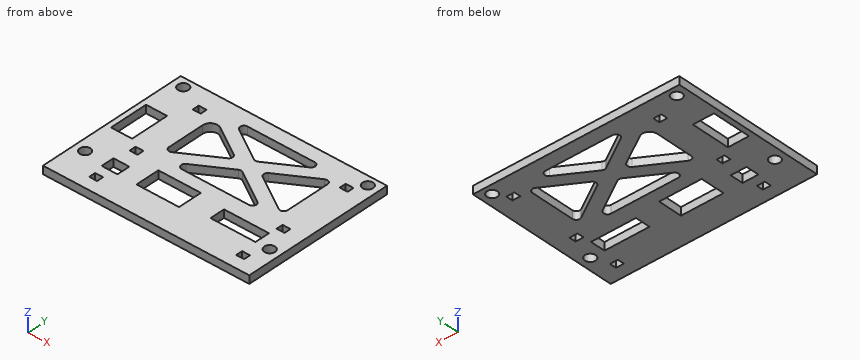
from build123d import *

# Parameters (mm, degrees)
SKETCH1_W              = 41.275
SKETCH1_H              = 25.4
SKETCH1_R              = 1.0541
SKETCH1_H_2            = 5.08
BOSS_EXTRUDE1_DEPTH    = 1.5875
ATTACHMENT_HOLES_REACH = 34.766
SKETCH3_W              = 1.5875
SKETCH3_H              = 1.3208
SKETCH2_W              = 8.509
SKETCH2_H              = 4.826
SKETCH2_W_2            = 4.22
SKETCH2_H_2            = 7.75
SKETCH2_W_3            = 3.175
SKETCH2_H_3            = 2.6162
SKETCH2_W_4            = 9
SKETCH2_H_4            = 2.985879982
CUT_EXTRUDE1_DEPTH     = 1.5875
FILLET8_R              = 0.762
FILLET9_R              = 1.524


with BuildPart() as part:
    # Sketch1 → Boss-Extrude1 (new body)
    # profile 1 of 2: a face of its own
    with BuildSketch(Plane.XY):
        with Locations((0, 12.7)):
            Rectangle(SKETCH1_W, SKETCH1_H)
        with Locations((-18.4658, 1.8415)):
            Circle(SKETCH1_R, mode=Mode.SUBTRACT)
        with Locations((18.4658, 1.8415)):
            Circle(SKETCH1_R, mode=Mode.SUBTRACT)
        with Locations((-18.4658, 23.5585)):
            Circle(SKETCH1_R, mode=Mode.SUBTRACT)
        with Locations((18.4658, 23.5585)):
            Circle(SKETCH1_R, mode=Mode.SUBTRACT)
    # profile 2 of 2: a face of its own
    with BuildSketch(Plane.XY):
        with Locations((0, -2.54)):
            Rectangle(SKETCH1_W, SKETCH1_H_2)
    extrude(amount=BOSS_EXTRUDE1_DEPTH)

    # Sketch3 → Attachment Holes (cut, up to next)
    with BuildSketch(Plane(origin=(0, 0, 0), x_dir=(-1, 0, 0), z_dir=(0, 0, -1)), mode=Mode.PRIVATE) as attachment_holes_sk1:
        with Locations((-16.54175, 20.992155968)):
            Rectangle(SKETCH3_W, SKETCH3_H)
    attachment_holes_tool1 = extrude(attachment_holes_sk1.sketch, amount=-ATTACHMENT_HOLES_REACH, mode=Mode.PRIVATE) & part.part
    # Sketch3 → Attachment Holes (cut, up to next)
    with BuildSketch(Plane(origin=(0, 0, 0), x_dir=(-1, 0, 0), z_dir=(0, 0, -1)), mode=Mode.PRIVATE) as attachment_holes_sk2:
        with Locations((-16.54175, 7.022155968)):
            Rectangle(SKETCH3_W, SKETCH3_H)
    attachment_holes_tool2 = extrude(attachment_holes_sk2.sketch, amount=-ATTACHMENT_HOLES_REACH, mode=Mode.PRIVATE) & part.part
    # Sketch3 → Attachment Holes (cut, up to next)
    with BuildSketch(Plane(origin=(0, 0, 0), x_dir=(-1, 0, 0), z_dir=(0, 0, -1)), mode=Mode.PRIVATE) as attachment_holes_sk3:
        with Locations((-16.54175, -1.918644032)):
            Rectangle(SKETCH3_W, SKETCH3_H)
    attachment_holes_tool3 = extrude(attachment_holes_sk3.sketch, amount=-ATTACHMENT_HOLES_REACH, mode=Mode.PRIVATE) & part.part
    # Sketch3 → Attachment Holes (cut, up to next)
    with BuildSketch(Plane(origin=(0, 0, 0), x_dir=(-1, 0, 0), z_dir=(0, 0, -1)), mode=Mode.PRIVATE) as attachment_holes_sk4:
        with Locations((12.85875, 20.992155968)):
            Rectangle(SKETCH3_W, SKETCH3_H)
    attachment_holes_tool4 = extrude(attachment_holes_sk4.sketch, amount=-ATTACHMENT_HOLES_REACH, mode=Mode.PRIVATE) & part.part
    # Sketch3 → Attachment Holes (cut, up to next)
    with BuildSketch(Plane(origin=(0, 0, 0), x_dir=(-1, 0, 0), z_dir=(0, 0, -1)), mode=Mode.PRIVATE) as attachment_holes_sk5:
        with Locations((12.85875, 7.022155968)):
            Rectangle(SKETCH3_W, SKETCH3_H)
    attachment_holes_tool5 = extrude(attachment_holes_sk5.sketch, amount=-ATTACHMENT_HOLES_REACH, mode=Mode.PRIVATE) & part.part
    # Sketch3 → Attachment Holes (cut, up to next)
    with BuildSketch(Plane(origin=(0, 0, 0), x_dir=(-1, 0, 0), z_dir=(0, 0, -1)), mode=Mode.PRIVATE) as attachment_holes_sk6:
        with Locations((12.85875, -1.918644032)):
            Rectangle(SKETCH3_W, SKETCH3_H)
    attachment_holes_tool6 = extrude(attachment_holes_sk6.sketch, amount=-ATTACHMENT_HOLES_REACH, mode=Mode.PRIVATE) & part.part
    add(attachment_holes_tool1.solids().sort_by_distance((16.54175, 20.992156, 0))[0], mode=Mode.SUBTRACT)
    add(attachment_holes_tool2.solids().sort_by_distance((16.54175, 7.022156, 0))[0], mode=Mode.SUBTRACT)
    add(attachment_holes_tool3.solids().sort_by_distance((16.54175, -1.918644, 0))[0], mode=Mode.SUBTRACT)
    add(attachment_holes_tool4.solids().sort_by_distance((-12.85875, 20.992156, 0))[0], mode=Mode.SUBTRACT)
    add(attachment_holes_tool5.solids().sort_by_distance((-12.85875, 7.022156, 0))[0], mode=Mode.SUBTRACT)
    add(attachment_holes_tool6.solids().sort_by_distance((-12.85875, -1.918644, 0))[0], mode=Mode.SUBTRACT)

    # Sketch2 → Cut-Extrude1 (cut)
    with BuildSketch(Plane.XY.offset(1.5875)):
        Polygon((11.409828794, 8.0735), (1.9685, 13.850842654), (-7.472828794, 8.0735), align=None)
        Polygon((13.843, 21.117092654), (4.401671206, 15.33975), (13.843, 9.562407346), align=None)
        Polygon((-7.472828794, 22.606), (1.9685, 16.828657346), (11.409828794, 22.606), align=None)
        Polygon((-0.464671206, 15.33975), (-9.906, 21.117092654), (-9.906, 9.562407346), align=None)
        with Locations((-2.8993, 3.1205)):
            Rectangle(SKETCH2_W, SKETCH2_H)
        with Locations((-17.4978, 12.709)):
            Rectangle(SKETCH2_W_2, SKETCH2_H_2)
        with Locations((-12.5513, 2.0156)):
            Rectangle(SKETCH2_W_3, SKETCH2_H_3)
        with Locations((11.1858, 3.267239991)):
            Rectangle(SKETCH2_W_4, SKETCH2_H_4)
    extrude(amount=-CUT_EXTRUDE1_DEPTH, mode=Mode.SUBTRACT)

    # Fillet8
    fillet8_edges = [part.edges().sort_by_distance(p)[0] for p in [
        (-7.472828794, 8.0735, 0.79375),
        (1.9685, 13.850842654, 0.79375),
        (11.409828794, 8.0735, 0.79375),
        (4.401671206, 15.33975, 0.79375),
        (13.843, 21.117092654, 0.79375),
        (13.843, 9.562407346, 0.79375),
        (1.9685, 16.828657346, 0.79375),
        (-7.472828794, 22.606, 0.79375),
        (11.409828794, 22.606, 0.79375),
        (-9.906, 9.562407346, 0.79375),
        (-0.464671206, 15.33975, 0.79375),
    ]]
    fillet(fillet8_edges, radius=FILLET8_R)

    # Fillet9
    fillet9_edges = [part.edges().sort_by_distance(p)[0] for p in [
        (-9.906, 21.117092654, 0.79375),
    ]]
    fillet(fillet9_edges, radius=FILLET9_R)


solid = part.part
Here's how the part is built. I have some questions about the finished solid (model axes, mm). Round coordinates to 2 decimals unless told otherwise and drop trailing zeros. Loops run counter-clockwise (first coordinate to the right, second up) from the corner with the lowest first, then second, coordinate; pieces in that order, holes last. Notation, with made-up numbers: M 11.25,-35.75 L 24.25,-35.75 A22 ccw 24.25,-8.75 Z; hole C 52.5,63 d9. An arc over 180 degrees is marked long. Write each question's results on one line, items separated by ' | '. Start each with the question number.
(1) Will these pins go through, and if not, where does the flat tip stop? P1, Ø1, axis at x = 4.5, y = 19.5, coming from the +Z side; P2, Ø3.5, axis at x = -18.47, y = 1.84, coming from the +Z side.
(2) I want a section at B-B (y = 7). Please give me the cut outline in (x, z) (1 decimal).
(3) If I drill on probe 1 along X at (y, z) = (23.5, 1.35); probe 2 along X at (y, z) = (6.5, 0.2) (1 decimal); probe 3 along X at (y, z) = (15, 1.2), over which ranges is the centre line in solid material (lowest first)? Write a range as from..to.
(4) I want a section at C-C (x = -12.5). Please give me the cut outline in (y, z), then the cut area to 3 significant figures.
(5) I want a section at A-A (x = 15). Please give me the cut outline in (y, z), then the cut area to 3 significant figures.
(6) I want a section at D-D (x = -2). Please give me the cut outline in (y, z).
Solved:
1) P1: passes through | P2: stops at z = 1.59
2) outline: M -20.6,0 L -13.7,0 L -13.7,1.6 L -20.6,1.6 Z; M -12.1,0 L 15.7,0 L 15.7,1.6 L -12.1,1.6 Z; M 17.3,0 L 20.6,0 L 20.6,1.6 L 17.3,1.6 Z
3) probe 1: x = -20.64..-19.52, -17.41..17.41, 19.52..20.64 | probe 2: x = -20.6..-13.7, -12.1..15.7, 17.3..20.6 | probe 3: x = -20.64..-19.61, -15.39..-9.91, -1.24..5.18, 13.84..20.64
4) outline: M -5.08,0 L -2.58,0 L -2.58,1.59 L -5.08,1.59 Z; M -1.26,0 L 0.71,0 L 0.71,1.59 L -1.26,1.59 Z; M 3.32,0 L 6.36,0 L 6.36,1.59 L 3.32,1.59 Z; M 7.68,0 L 20.33,0 L 20.33,1.59 L 7.68,1.59 Z; M 21.65,0 L 25.4,0 L 25.4,1.59 L 21.65,1.59 Z | area: 37.9 mm²
5) outline: M -5.08,0 L 1.77,0 L 1.77,1.59 L -5.08,1.59 Z; M 4.76,0 L 25.4,0 L 25.4,1.59 L 4.76,1.59 Z | area: 43.6 mm²
6) outline: M -5.08,0 L 0.71,0 L 0.71,1.59 L -5.08,1.59 Z; M 5.53,0 L 8.07,0 L 8.07,1.59 L 5.53,1.59 Z; M 11.42,0 L 14.4,0 L 14.4,1.59 L 11.42,1.59 Z; M 16.28,0 L 19.26,0 L 19.26,1.59 L 16.28,1.59 Z; M 22.61,0 L 25.4,0 L 25.4,1.59 L 22.61,1.59 Z
